Read the model definition and answer for the solid it produces. Units are mm, in the model's axes. A direction names the side the tool comes from. Round coordinates to 2 decimals unless told otherwise and drop trailing zeros. Order: outer loops, then holes, each group sorted by start corner. A loop starts at its lowest first (then second) coordinate and runs counter-clockwise, first axis right, second up.
from build123d import *

# Parameters (mm, degrees)
F3_D = 16.66748


with BuildPart() as f1:
    # F0 (on Front) → F1 (revolve)
    with BuildSketch(Plane.XZ):
        with BuildLine():
            Line((-44.831, -6.7267071241), (-53.721, -6.7267071241))
            Line((-53.721, -6.7267071241), (-53.721, -20.0617071241))
            Line((-53.721, -20.0617071241), (0, -20.0617071241))
            Line((0, -20.0617071241), (0, 17.7842928759))
            Line((0, 17.7842928759), (-13.716, 17.7842928759))
            Line((-13.716, 17.7842928759), (-13.716, 7.6767612798))
            Line((-13.716, 7.6767612798), (-20.32, 7.6767612798))
            ThreePointArc((-20.32, 7.6767612798), (-33.1625249148, 5.7126824661), (-44.831, 0))
            Line((-44.831, 0), (-44.831, -6.7267071241))
        make_face()
    revolve(axis=Axis((0, 0, -1.1387071241), (0, 0, 1)))

    # F3 (through all)
    with Locations(Plane.XY.offset(17.7842928759)):
        with Locations((0, 0)):
            Hole(F3_D / 2)


solid = f1.part
Q1. A cutting plane is placed at A-A, the plane z = -15.5. Give the vertices of the cut face in (x, y).
Outcome:
outline: circle Ø107.44 at (0, 0); hole circle Ø16.67 at (0, 0)
Q2. For faces 1 (the face through (6, 6, 17.784)), 2 (the face through (-42.76, -13.47, -3.41)), determine the directions among +Z, -Z, +X, -X, +Y, -Y from which every point of the face is accessible in a straight line to the end or side of a thin tool.
Outcome:
face 1: +Z, +X, -X, +Y, -Y
face 2: +Z
Q3. Flat-ended cylindrical pins translate along their axes: pin 1 (4 mm diameter, centred on y = 9, z = 5.5, fed in from +X); pin 2 (13.5 mm diameter, centred on x = 0, y = 0, fed in from +Z); pin 3 (8 mm diameter, centred on y = 0, z = 12, fed in from +X); pin 4 (1 mm diameter, centred on y = -18, z = -3.5, fed in from -X). Find the tip coordinate at first contact, or state that the pin passes through.
Outcome:
pin 1: stops at x = 37.77
pin 2: passes through
pin 3: stops at x = 13.72
pin 4: stops at x = -41.27
Q4. Straight lines are drawn through the part: probe 1 along Y at (x, z) = (0, 10); probe 2 along Y at (x, z) = (0, -10); probe 3 along Z at (x, y) = (13, 11). For each, find the intervals that lie inside material, in ascending order.
Outcome:
probe 1: y = -13.72 to -8.33, 8.33 to 13.72
probe 2: y = -53.72 to -8.33, 8.33 to 53.72
probe 3: z = -20.06 to 7.68
Q5. For a pull along X with two mould halves and no side action, classify faces 3 (the face through (6.993, -53.264, -13.488)), 4 (the face through (8.326, 0.366, -1.404)), 5 (the face through (1, 11, -20.062)) as released by +X, released by -X, zero draft, split by the parting line, or undercut.
Outcome:
face 3: split by the parting line
face 4: undercut
face 5: zero draft
Q6. A cutting plane is placed at B-B, the plane z = -5. Give the vertices of the cut face in (x, y).
Outcome:
outline: circle Ø89.66 at (0, 0); hole circle Ø16.67 at (0, 0)
